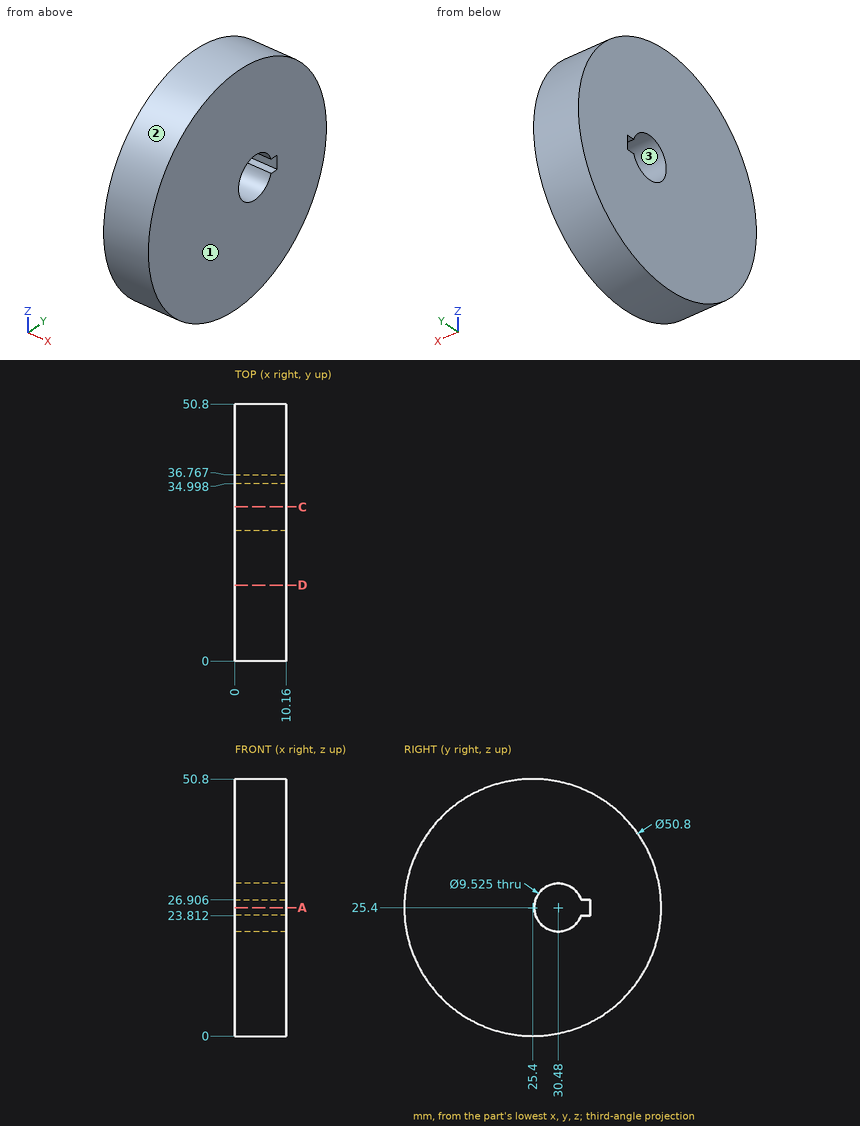
Answer from the drawing. Dimensions are ordinates in mm from the lowest x, y and z of the part. Round coordinates to 2 decimals unless told otherwise and drop trailing zeros. Loops run counter-clockwise (first coordinate to the right, second up) from the corner with the lowest first, then second, coordinate; pieces in that order, holes last. Notation, with made-up numbers: (34.25, -33) - (46.25, -33) arc R20 ccw to (46.25, 4) - close; hole circle Ø3 at (71.5, -22.5). An arc over 180 degrees is marked (long way). Return JSON: item names as keys, results as strings. Group by question number.
1. The mould has two halves that part along Y. Classify the marked faces 1, 2 and 3: pulls with the +Y half, pulls with the -Y half, needs draft (parallel to the pull), parting line crosses it, or undercut.
2. The part is cut by section D-D on y = 15. Determine the outline of the cut face in (x, z), then the cut area to 3 significant figures.
3. Each of these flat-tipped pins is pushed along its axis until it touches: P1, Ø1, axis at x = 4, y = 17, coming from the +Z side; P2, Ø5, axis at x = 5.5, z = 16.5, coming from the -Y side; P3, Ø3.5, axis at x = 6, z = 25.5, coming from the -Y side; P4, Ø8.5, axis at y = 30.48, z = 25.4, coming from the +X side. Where does it stop, or does it pass through?
4. The part is cut by section C-C on y = 30.48. Determine the outline of the cut face in (x, z).
5. Consider probe 1 along Y at (x, z) = (2.25, 25.4); probe 2 along Y at (x, z) = (9.75, 29) (1 decimal); probe 3 along Z at (x, y) = (8, 27.5) (1 decimal). Determine where each line is inside the solid, lowest interval first.
6. The part is cut by section A-A on z = 25.4. Determine the outline of the cut face in (x, y), then the cut area to 3 significant figures.
Resolved:
{
 "1": {"face 1": "needs draft", "face 2": "parting line crosses it", "face 3": "undercut"},
 "2": {"outline": "(0, 2.23) - (10.16, 2.23) - (10.16, 48.57) - (0, 48.57) - close", "area": "471 mm²"},
 "3": {"P1": "stops at z = 49.54", "P2": "stops at y = 0.82", "P3": "stops at y = 0", "P4": "passes through"},
 "4": {"outline": "(0, 0.51) - (10.16, 0.51) - (10.16, 20.64) - (0, 20.64) - close; (0, 30.16) - (10.16, 30.16) - (10.16, 50.29) - (0, 50.29) - close"},
 "5": {"probe 1": "y = 0 to 25.72, 36.77 to 50.8", "probe 2": "y = 0.3 to 27.4, 33.6 to 50.5", "probe 3": "z = 0.1 to 21.7, 29.1 to 50.7"},
 "6": {"outline": "(0, 0) - (10.16, 0) - (10.16, 25.72) - (0, 25.72) - close; (0, 36.77) - (10.16, 36.77) - (10.16, 50.8) - (0, 50.8) - close", "area": "404 mm²"}
}
